Could you check a few things on this model? Use its own coordinates, in mm. Give positions to 0.01 mm unless a question says otherwise; leave off trailing zeros. Order: outer loops, then holes, each group sorted by start corner. A loop starts at its lowest first (then second) coordinate and runs counter-clockwise, first axis right, second up. Notation, with made-up numbers: M 89,10 L 141,10 A16 cw 141,24 Z; hole C 50.25,20.25 d2. An arc over 180 degrees is marked long. Use a Markdown table: item, result. Add a question column.
Item 1: Suppose I cut it at A-A on x = 45. Write out the boundary of the cut face in (y, z).
Item 2: Suppose I cut it at C-C on x = 10. Write out the boundary of the cut face in (y, z), plus the area to 3 significant figures.
Item 3: If we mould it in two halves opening along Z, with no side actions, what happens to faces 1 (the face through (58, 5, 0)), 2 (the face through (100, 5, 17)), 3 (the face through (9.74, 5.07, 20.517))? For each: released by +Z, released by -Z, zero draft, split by the parting line, or undercut.
Item 4: If I drill on L1, parallel to Z at x = 45, y = 6.5; L2, parallel to Z at x = 90, y = 6.25; L3, parallel to Z at x = 10, y = 5.5, over which ranges is the centre line in solid material (lowest first)? Write a range as from..to.
Item 5: Suppose I cut it at D-D on z = 12.5. Write out the boundary of the cut face in (x, y).
Item 6: Suppose I cut it at B-B on y = 5.5. Count the separate pieces of the cut face and the enclosed holes in it, plus the area to 3 significant figures.
Autodesk Inventor part; units mm, degrees
ref_plane "작업 평면1" through (50, 0, 0) normal (-1, 0, 0) x (0, 0, 1)
ref_plane "작업 평면2" through (65, 40, 45) normal (0, 1, 0) x (1, 0, 0)
ref_plane "작업 평면3" through (50, 0, 0) normal (1, 0, 0) x (0, 0, -1)
sketch "스케치1" plane through (0, 0, 0) normal (0, 0, 1) x (1, 0, 0)
  line L0 (0, 0) -> (100, 0)
  line L1 (100, 0) -> (100, 10)
  line L2 (100, 10) -> (0, 10)
  line L3 (0, 10) -> (0, 0)
  dimension "d0" = 100
  dimension "d1" = 10
extrude "돌출1" add sketch "스케치1" along normal blind 35
sketch "스케치3" plane through (0, 0, 0) normal (0, -1, 0) x (1, 0, 0)
  line L0 (0, 0) -> (100, 0)
  line L1 (100, 0) -> (100, 35)
  line L2 (0, 35) -> (100, 35)
  line L3 (0, 0) -> (0, 35)
  circle A0 centre (90, 17.5) radius 7.5
  point P0 (15, 17.5)
  point P1 (100, 17.5)
  dimension "d8" = 15
  dimension "d12" = 10
extrude "돌출3" cut sketch "스케치3" against normal through all contours A0
ref_plane "작업 평면1" through (50, 0, 0) normal (-1, 0, 0) x (0, 0, 1)
ref_plane "작업 평면2" through (65, 40, 45) normal (0, 1, 0) x (1, 0, 0)
ref_plane "작업 평면3" through (50, 0, 0) normal (1, 0, 0) x (0, 0, -1)
sketch "스케치4" plane through (0, 10, 0) normal (0, 1, 0) x (1, 0, 0)
  circle A0 centre (90, -17.5) radius 7.5
  line L0 (100, 0) -> (0, 0)
  line L1 (0, 0) -> (0, -35)
  line L2 (100, -35) -> (0, -35)
  line L3 (100, 0) -> (100, -35)
  circle A1 centre (45, -17.5) radius 2.6
  circle A2 centre (55, -17.5) radius 2.6
  line L4 (100, 0) -> (0, 0)
  point P0 (50, 0)
  point P1 (50, 0)
  point P2 (100, -17.5)
  dimension "d16" = 5.2
  dimension "d17" = 5.2
  dimension "d18" = 10
  dimension "d19" = 5
extrude "돌출4" cut sketch "스케치4" against normal through all contours A1 | A2
sketch "스케치5" plane through (0, 10, 0) normal (0, 1, 0) x (1, 0, 0)
  circle A0 centre (10, -12.5) radius 2
  circle A1 centre (10, -22.5) radius 2
  line L0 (0, 0) -> (0, -35)
  point P0 (0, -17.5)
  dimension "d20" = 4
  dimension "d21" = 4
  dimension "d22" = 10
  dimension "d23" = 5
  dimension "d24" = 10
extrude "돌출5" cut sketch "스케치5" against normal through all
fillet "모깎기1" radius 17.5 2 edges at (0, 5, 0) (0, 5, 35)
properties part number "다리-2"
Findings below:
| question | item | result |
|---|---|---|
| 1 | outline | M 0,0 L 10,0 L 10,14.9 L 0,14.9 Z; M 0,20.1 L 10,20.1 L 10,35 L 0,35 Z |
| 2 | outline | M 0,1.69 L 10,1.69 L 10,10.5 L 0,10.5 Z; M 0,14.5 L 10,14.5 L 10,20.5 L 0,20.5 Z; M 0,24.5 L 10,24.5 L 10,33.31 L 0,33.31 Z |
| 2 | area | 236 mm^2 |
| 3 | face 1 | released by -Z |
| 3 | face 2 | zero draft |
| 3 | face 3 | undercut |
| 4 | L1 | z = 0..14.9, 20.1..35 |
| 4 | L2 | z = 0..10, 25..35 |
| 4 | L3 | z = 1.69..10.5, 14.5..20.5, 24.5..33.31 |
| 5 | outline | M 0.73,0 L 8,0 L 8,10 L 0.73,10 Z; M 12,0 L 84.41,0 L 84.41,10 L 12,10 Z; M 95.59,0 L 100,0 L 100,10 L 95.59,10 Z |
| 6 | separate pieces | 1 |
| 6 | enclosed holes | 5 |
| 6 | area | 3,120 mm^2 |
